Can you work these out from the model? Positions are in its coordinate system, mm. Face numbers are marked on the shaded views. A direction names the side the tool comes from. Round coordinates to 2 decimals unless told otherwise and drop trailing zeros. Loops run counter-clockwise (first coordinate to the right, second up) from the corner with the lowest first, then second, coordinate; pieces in that order, holes last. Notation, with made-up numbers: M 62,66.5 L 68,66.5 A21 ccw 68,94.5 Z; hole C 47.25,88 d6. An arc over 180 degrees is marked long. Return JSON: item names as keys, results as strings.
```python
from build123d import *

# Parameters (mm, degrees)
BOSS_EXTRUDE1_DEPTH = 100
BOSS_EXTRUDE2_DEPTH = 5


with BuildPart() as part:
    # Sketch1 → Boss-Extrude1 (new body)
    with BuildSketch(Plane(origin=(0, 0, 0), x_dir=(1, 0, 0), z_dir=(0, 1, 0))):
        with BuildLine():
            Line((-113.861275844, 23.426394533), (-103.861275844, 23.426394533))
            Line((-103.861275844, 23.426394533), (-103.861275844, 72.756738269))
            ThreePointArc((-103.861275844, 72.756738269), (-38.861275844, -1.573605467), (-103.861275844, -75.903949204))
            Line((-103.861275844, -75.903949204), (-103.861275844, -26.573605467))
            Line((-103.861275844, -26.573605467), (-113.861275844, -26.573605467))
            Line((-113.861275844, -26.573605467), (-113.861275844, 23.426394533))
        make_face()
    extrude(amount=BOSS_EXTRUDE1_DEPTH)

    # Sketch2 → Boss-Extrude2 (add, symmetric)
    with BuildSketch(Plane(origin=(0, 50, 0), x_dir=(1, 0, 0), z_dir=(0, 1, 0))):
        with BuildLine():
            Line((-103.861275844, -75.903949204), (-103.861275844, -81.787530662))
            ThreePointArc((-103.861275844, -81.787530662), (-33.026420768, -1.573605467), (-103.861275844, 78.640319727))
            Line((-103.861275844, 78.640319727), (-103.861275844, 72.756738269))
            ThreePointArc((-103.861275844, 72.756738269), (-38.861275844, -1.573605467), (-103.861275844, -75.903949204))
        make_face()
    extrude(amount=BOSS_EXTRUDE2_DEPTH, both=True)


solid = part.part
```
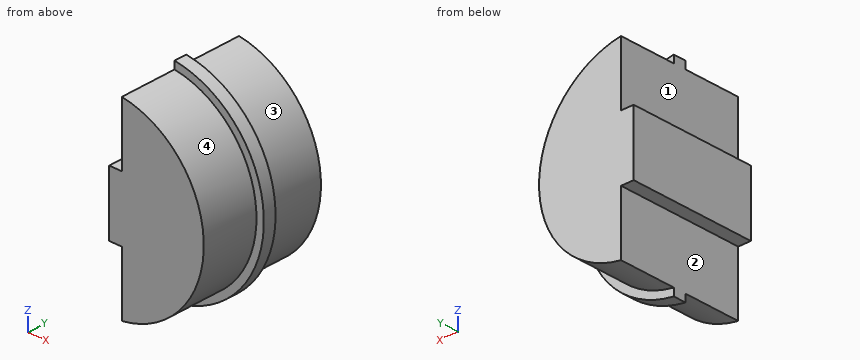
Q1. Suppose I cut it at B-B, the plane x = -65. Please give me the cut outline in (y, z).
Results:
{"outline": "M 0,-55.33 L 45,-55.33 L 45,-62.82 L 55,-62.82 L 55,-55.33 L 100,-55.33 L 100,58.47 L 55,58.47 L 55,65.97 L 45,65.97 L 45,58.47 L 0,58.47 Z"}
Q2. If I drill on line 1 along Z through (x, y) = (-70.5, 49); line 2 along Z through (x, y) = (-82, 59.5); line 3 along X through (y, z) = (65.5, 15.5), over which ranges is the centre line in solid material (lowest first)?
Results:
{"line 1": "z = -66.65 to 69.79", "line 2": "z = -66.32 to 69.47", "line 3": "x = -113.86 to -40.17"}
Q3. On a 3-axis mill with a long thin cutter (end or side, diameter ignored), from which of +Z, -Z, +X, -X, +Y, -Y can I reach the whole of each face in a straight line? I mean the marked faces 1, 2, 3 and 4. Say none if no direction works.
Results:
{"face 1": "+Z, -X, +Y, -Y", "face 2": "-Z, -X, +Y, -Y", "face 3": "+X, +Y", "face 4": "+X, -Y"}
Q4. Suppose I cut it at A-A, the plane y = 28.5. Please give me the cut outline in (x, z).
Results:
{"outline": "M -113.86,-23.43 L -103.86,-23.43 L -103.86,-72.76 A75 ccw -103.86,75.9 L -103.86,26.57 L -113.86,26.57 Z"}
Q5. Suppose I cut it at C-C, the plane z = 46. Please give me the cut outline in (x, y), plus the area to 3 significant figures.
Results:
{"outline": "M -103.86,0 L -53.44,0 L -53.44,45 L -46.33,45 L -46.33,55 L -53.44,55 L -53.44,100 L -103.86,100 Z", "area": "5,110 mm2"}
Q6. I'm going to push flat-ended pins straight in: pin 1 Ø5 at (x, y) = (-111, 26) entering from +Z; pin 2 Ø2 at (y, z) = (69, 62.5) entering from -X; pin 3 Ø5 at (y, z) = (34.5, -26.5) entering from +X. Where does each tip first touch, or does it pass through?
Results:
{"pin 1": "stops at z = 26.57", "pin 2": "stops at x = -103.86", "pin 3": "stops at x = -43.36"}
Q7. Suppose I cut it at D-D, the plane z = -35. Please give me the cut outline in (x, y), plus the area to 3 significant figures.
Results:
{"outline": "M -103.86,0 L -48.38,0 L -48.38,45 L -41.77,45 L -41.77,55 L -48.38,55 L -48.38,100 L -103.86,100 Z", "area": "5,610 mm2"}
